```python
from build123d import *

# Parameters (mm, degrees)
F0_R     = 5
F1_DEPTH = 5
F3_DEPTH = 25


with BuildPart() as f1:
    # F0 (on Top) → F1 (new body)
    with BuildSketch(Plane.XY):
        Polygon((-7.5, 70), (-14.5, 70), (-17.5, 0), (22.5, 0), (22.5, 15), (17.5, 15), (17.5, 45), (22.5, 45), (22.5, 70), (12.5, 70), (12.5, 75), (-7.5, 75), align=None)
        with Locations((0, 33)):
            Circle(F0_R, mode=Mode.SUBTRACT)
    extrude(amount=F1_DEPTH)

    # F2 (on face) → F3 (cut)
    with BuildSketch(Plane.XY.offset(5)):
        Polygon((17.5, 15), (10.5, 0), (22.5, 0), (22.5, 15), align=None)
    extrude(amount=-F3_DEPTH, mode=Mode.SUBTRACT)


solid = f1.part
```
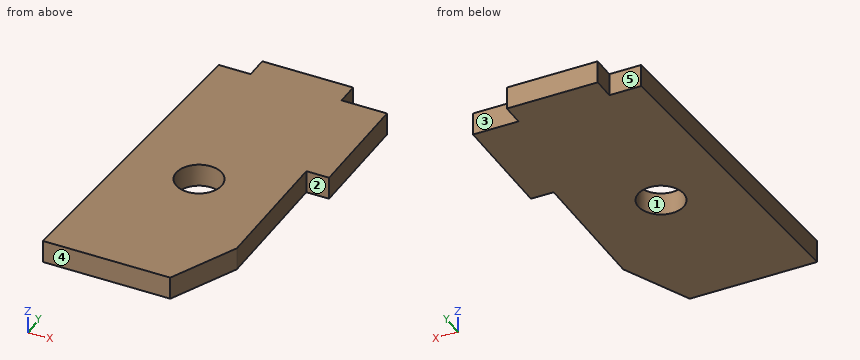
Verification items for the finished model (mm, model axes). Face numbers are marked on the shaded views. A direction names the side the tool comes from. Give positions to 0.01 mm unless a question says otherwise; leave off trailing zeros. Order: outer loops, then holes, each group sorted by start corner. A loop starts at its lowest first (then second) coordinate and runs counter-clockwise, first axis right, second up. Notation, with made-up numbers: M 37,-25.5 L 96,-25.5 A25 ccw 96,9.5 Z; hole C 48.5,88 d6. An arc over 180 degrees is marked long. Answer in a Markdown table with one row per item. Add a question column.
Item 1: Section check B-B, the plane z = 1.3. Enter the section's corners in (x, y), and give its area (3 significant figures).
Item 2: Section check C-C, the plane y = 33. Enter the section's corners in (x, z), and give its area (3 significant figures).
Item 3: Section check D-D, the plane x = -9. Enter the section's corners in (y, z).
Item 4: Tool access check on the marked faces 4 and 5. Record the directions out of +Z, -Z, +X, -X, +Y, -Y that give a thin tool (end or side, any length) a straight path to the whole face; none if there is none.
Item 5: Scan lines: probe 1 along Y at (x, z) = (0, 3.25); probe 2 along Y at (x, z) = (-9, 3.85); probe 3 along X at (y, z) = (34.5, 0.5). Record each from-to range of solid material in increasing order. Write a range as from..to.
Item 6: Section check A-A, the plane x = 0. Enter the section's corners in (y, z).
Item 7: Gauge pin test, flat ends, axial feed: pin 1 (2.5 mm diameter, centred on y = 73.5, z = 1.5, fed in from +X); pin 2 (1.5 mm diameter, centred on y = 36, z = 1.5, fed in from +X); pin 3 (2.5 mm diameter, centred on x = -11.5, z = 3.5, fed in from +Y). Record the tip position at first contact, or that the pin passes through.
Item 8: Mould release check, pull along Y, two halves, no side actions. Record for the marked faces 1, 2 and 3: released by +Y, released by -Y, zero draft, split by the parting line, or undercut.
Filled sheet:
| question | item | result |
|---|---|---|
| 1 | outline | M -17.5,0 L 10.5,0 L 17.5,15 L 17.5,45 L 22.5,45 L 22.5,70 L 12.5,70 L 12.5,75 L -7.5,75 L -7.5,70 L -14.5,70 Z; hole C 0,33 d10 |
| 1 | area | 2,440 mm^2 |
| 2 | outline | M -16.09,0 L -5,0 L -5,5 L -16.09,5 Z; M 5,0 L 17.5,0 L 17.5,5 L 5,5 Z |
| 2 | area | 118 mm^2 |
| 3 | outline | M 0,0 L 70,0 L 70,5 L 0,5 Z |
| 4 | face 4 | +Z, -Z, +X, -X, -Y |
| 4 | face 5 | +Z, -Z, -X, +Y |
| 5 | probe 1 | y = 0..28, 38..75 |
| 5 | probe 2 | y = 0..70 |
| 5 | probe 3 | x = -16.02..-4.77, 4.77..17.5 |
| 6 | outline | M 0,0 L 28,0 L 28,5 L 0,5 Z; M 38,0 L 75,0 L 75,5 L 38,5 Z |
| 7 | pin 1 | stops at x = 12.5 |
| 7 | pin 2 | stops at x = 17.5 |
| 7 | pin 3 | stops at y = 70 |
| 8 | face 1 | undercut |
| 8 | face 2 | released by -Y |
| 8 | face 3 | released by +Y |
